Answer from the drawing. Dimensions are ordinates in mm from the lowest x, y and z of the part. A direction names the side the tool comes from. Round coordinates to 2 decimals unless told otherwise and drop trailing zeros. Loops run counter-clockwise (first coordinate to the right, second up) from the corner with the lowest first, then second, coordinate; pieces in that order, holes last. Notation, with made-up numbers: (86, 33) - (142, 33) arc R13 ccw to (142, 37) - close; hole circle Ø5 at (86.5, 52.25). An arc over 180 degrees is marked (long way). Answer as CSV lines item,"result". Start each with the question number.
Q1. Section A-A on z = 4 is taken. Count the separate pieces of the cut face and the enclosed holes in it, then the cut area to 3 significant figures.
Q2. Straight lines are drawn through the part: L1, parallel to X at y = 2, z = 3.5 (1 decimal); L2, parallel to Y at x = 21, z = 4.25 (1 decimal); L3, parallel to Y at x = 7, z = 4.5 (1 decimal). For each, find the intervals that lie inside material, in ascending order. Write a range as [from, to].
Q3. The mould has two halves that part along Z. Classify the marked faces 1, 2, 3 and 4: +Z half, -Z half, draft (parallel to the pull), parting line (faces both ways), or undercut.
Q4. For the marked faces 5 and 6, determine the directions among +Z, -Z, +X, -X, +Y, -Y from which every point of the face is accessible in a straight line to the end or side of a thin tool.
Q5. Section D-D on y = 27.5 is taken. Write down the section's boundary in (x, z) (1 decimal).
Q6. Each of these flat-tipped pins is pushed along its axis until it touches: pin 1 Ø1.5 at (x, z) = (20, 6) entering from +Y (1 decimal); pin 2 Ø3 at (y, z) = (14.5, 3) entering from +X; pin 3 Ø5.5 at (x, z) = (30.87, 4.76) entering from +Y (1 decimal). Where does it stop, or does it pass through?
Q7. Section C-C on x = 10.5 is taken. Write down the section's boundary in (y, z) (1 decimal), then the cut area to 3 significant figures.
Q8. Section B-B on y = 7 is taken. Write down the section's boundary in (x, z) (1 decimal).
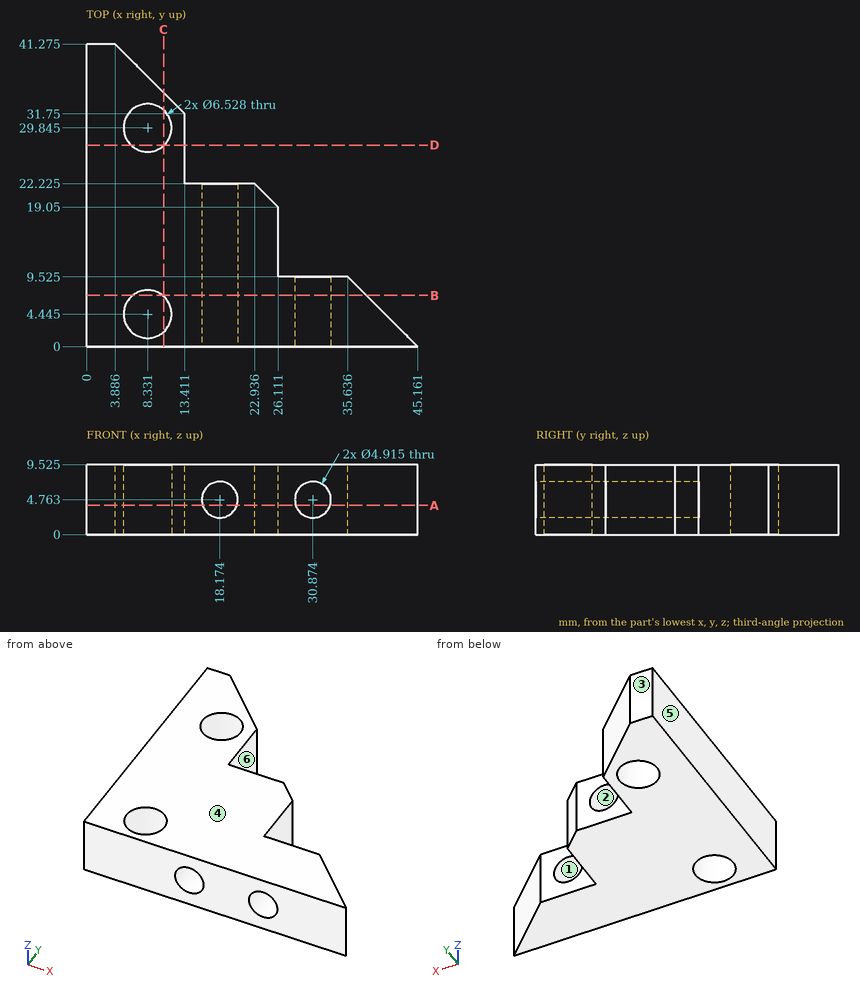
Findings:
1,separate pieces,"3"
1,enclosed holes,"2"
1,area,"706 mm^2"
2,L1,"x = [0, 6.2], [10.5, 16.1], [20.3, 28.8], [33, 43.2]"
2,L2,"y = [0, 22.2]"
2,L3,"y = [0, 1.5], [7.4, 26.9], [32.8, 38.2]"
3,face 1,"undercut"
3,face 2,"undercut"
3,face 3,"draft"
3,face 4,"+Z half"
4,face 5,"+Z, -Z, -X, +Y, -Y"
4,face 6,"+Z, -Z, +X, +Y"
5,outline,"(0, 0) - (6.1, 0) - (6.1, 9.5) - (0, 9.5) - close; (10.6, 0) - (13.4, 0) - (13.4, 9.5) - (10.6, 9.5) - close"
6,pin 1,"stops at y = 22.2"
6,pin 2,"stops at x = 26.11"
6,pin 3,"stops at y = 9.5"
7,outline,"(0, 0) - (2, 0) - (2, 9.5) - (0, 9.5) - close; (6.9, 0) - (27.4, 0) - (27.4, 9.5) - (6.9, 9.5) - close; (32.3, 0) - (34.7, 0) - (34.7, 9.5) - (32.3, 9.5) - close"
7,area,"237 mm^2"
8,outline,"(0, 0) - (6.3, 0) - (6.3, 9.5) - (0, 9.5) - close; (10.4, 0) - (38.2, 0) - (38.2, 9.5) - (10.4, 9.5) - close; hole circle Ø4.9 at (18.2, 4.8); hole circle Ø4.9 at (30.9, 4.8)"
